For this review, take the finished solid that the model builds, in its own axes (mm). A direction names the side the tool comes from. Give positions to 0.01 mm unless a question says otherwise; leave off trailing zeros. Loops run counter-clockwise (first coordinate to the right, second up) from the corner with the lowest first, then second, coordinate; pieces in that order, holes last. Notation, with made-up numbers: (40, 34.5) - (51, 34.5) arc R33 cw to (51, 68.5) - close; hole circle Ø11 at (33, -9). An arc over 180 degrees is marked (long way). Use CSV: the item, a comma, the result in double quotes. Start each with the question number.
1. For faces 5 (the flat face through (0, -19, 6)), 6 (the cylindrical face through (6.79, -26.58, 14.1)), 7 (the flat face through (2, -15.24, 9)), list the 3-axis set-ups (+Z, -Z, +X, -X, +Y, -Y) from which the entire face can be reached by the end or side of a thin tool; tool diameter is ignored.
2. Mouldability with a two-part tool opening along Y and no side actions: class faces 1 (the flat face through (4, -30.48, 4)), 2 (the flat face through (8, -15, 0)), 3 (the flat face through (8, 0, 1)), 4 (the cylindrical face through (10.65, -6.67, 1.29)) as pulls with the +Y half, pulls with the -Y half, needs draft (parallel to the pull), parting line crosses it, or undercut.
3. Take a section at B-B on x = 7.62. Give the boundary of the cut face in (y, z) (3 decimals).
4. Take a section at D-D on y = -22.86. Give the boundary of the cut face in (x, z), plus the area to 3 significant figures.
5. Wall thickness on line 1 (X direction, y = -22.86, z = 14); line 2 (Y direction, x = 7.62, z = 14.15); line 3 (Y direction, x = 7.62, z = 1.8) (3 decimals): over which ranges is each line inside the solid? List them lowest first.
6. For pin 1 (4.5 mm diameter, centred on x = 7, y = -8.5, fed in from +Z), flat-tipped, find the tip position at first contact; note if it passes through.
7. Take a section at A-A on y = -7.62. Give the boundary of the cut face in (x, z) (3 decimals), plus the area to 3 significant figures.
8. Take a section at C-C on z = 8.89. Give the boundary of the cut face in (x, y), plus the area to 3 significant figures.
```python
from build123d import *

# Parameters (mm, degrees)
F0_W     = 15.24
F0_H     = 30.48
F1_DEPTH = 2.54
F2_W     = 15.24
F2_H     = 15.24
F3_DEPTH = 12.7
F4_R     = 3.175
F5_DEPTH = 25.4
F6_R     = 5.08
F7_DEPTH = 25.4
F8_R     = 3.81
F9_DEPTH = 3.556


with BuildPart() as f1:
    # F0 (on Top) → F1 (new body)
    with BuildSketch(Plane.XY):
        with Locations((7.62, -15.24)):
            Rectangle(F0_W, F0_H)
    extrude(amount=F1_DEPTH)

    # F2 (on face) → F3 (join)
    with BuildSketch(Plane.XY.offset(2.54)):
        with Locations((7.62, -22.86)):
            Rectangle(F2_W, F2_H)
    extrude(amount=F3_DEPTH)

    # F4 (on face) → F5 (cut)
    with BuildSketch(Plane.XY.offset(2.54)):
        with Locations((7.62, -7.62)):
            Circle(F4_R)
    extrude(amount=-F5_DEPTH, mode=Mode.SUBTRACT)

    # F6 (on face) → F7 (cut)
    with BuildSketch(Plane(origin=(0, -15.24, 0), x_dir=(-1, 0, 0), z_dir=(0, 1, 0))):
        with Locations((-7.62, 8.89)):
            Circle(F6_R)
    extrude(amount=-F7_DEPTH, mode=Mode.SUBTRACT)

    # F8 (on face) → F9 (cut)
    with BuildSketch(Plane.XY.offset(15.24)):
        with Locations((7.62, -22.86)):
            Circle(F8_R)
    extrude(amount=-F9_DEPTH, mode=Mode.SUBTRACT)


solid = f1.part
```
Check result:
1,face 5,"+Z, -Z, -X, +Y, -Y"
1,face 6,"+Z"
1,face 7,"+Z, +X, -X, +Y"
2,face 1,"pulls with the -Y half"
2,face 2,"needs draft"
2,face 3,"pulls with the +Y half"
2,face 4,"undercut"
3,outline,"(-30.48, 0) - (-10.795, 0) - (-10.795, 2.54) - (-15.24, 2.54) - (-15.24, 3.81) - (-30.48, 3.81) - close; (-30.48, 13.97) - (-26.67, 13.97) - (-26.67, 15.24) - (-30.48, 15.24) - close; (-19.05, 13.97) - (-15.24, 13.97) - (-15.24, 15.24) - (-19.05, 15.24) - close; (-4.445, 0) - (0, 0) - (0, 2.54) - (-4.445, 2.54) - close"
4,outline,"(0, 0) - (15.24, 0) - (15.24, 15.24) - (11.43, 15.24) - (11.43, 12.25) arc R5.08 cw (long way) to (3.81, 12.25) - (3.81, 15.24) - (0, 15.24) - close"
4,area,"137 mm²"
5,line 1,"x = 0 to 3.81, 11.43 to 15.24"
5,line 2,"y = -30.48 to -26.67, -19.05 to -15.24"
5,line 3,"y = -30.48 to -10.795, -4.445 to 0"
6,pin 1,"stops at z = 2.54"
7,outline,"(0, 0) - (4.445, 0) - (4.445, 2.54) - (0, 2.54) - close; (10.795, 0) - (15.24, 0) - (15.24, 2.54) - (10.795, 2.54) - close"
7,area,"22.6 mm²"
8,outline,"(0, -30.48) - (2.54, -30.48) - (2.54, -15.24) - (0, -15.24) - close; (12.7, -30.48) - (15.24, -30.48) - (15.24, -15.24) - (12.7, -15.24) - close"
8,area,"77.4 mm²"
